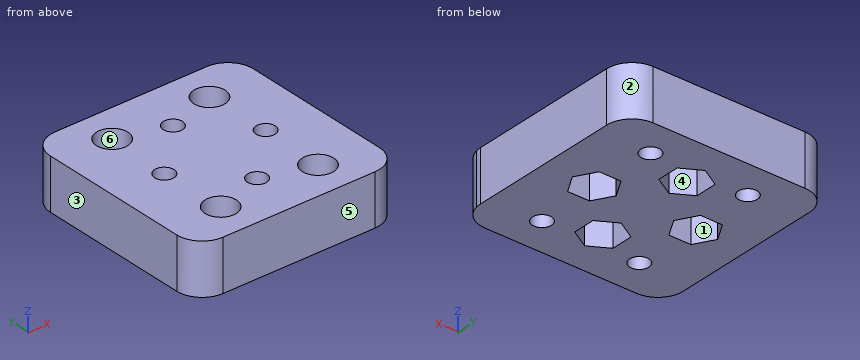
```python
from build123d import *

# Parameters (mm, degrees)
SKETCH1_W           = 50.8
SKETCH1_H           = 50.8
SKETCH1_R           = 2.413
BOSS_EXTRUDE1_DEPTH = 12.7
SKETCH2_R           = 2.413
CUT_EXTRUDE2_DEPTH  = 12.7
SKETCH7_R           = 2.413
CUT_EXTRUDE5_DEPTH  = 6.35
CUT_EXTRUDE6_DEPTH  = 73.955945611
SKETCH13_R          = 3.937
CUT_EXTRUDE7_DEPTH  = 4.826


with BuildPart() as part:
    # Sketch1 → Boss-Extrude1 (new body)
    with BuildSketch(Plane.XY):
        with Locations((25.4, -25.4)):
            Rectangle(SKETCH1_W, SKETCH1_H)
        with Locations((13.219909227, -9.017)):
            Circle(SKETCH1_R, mode=Mode.SUBTRACT)
        with Locations((37.603909227, -9.017)):
            Circle(SKETCH1_R, mode=Mode.SUBTRACT)
        with Locations((13.219909227, -41.783)):
            Circle(SKETCH1_R, mode=Mode.SUBTRACT)
        with Locations((37.603909227, -41.783)):
            Circle(SKETCH1_R, mode=Mode.SUBTRACT)
    extrude(amount=BOSS_EXTRUDE1_DEPTH)

    # Sketch2 → Cut-Extrude2 (cut)
    with BuildSketch(Plane(origin=(0, 0, 0), x_dir=(-1, 0, 0), z_dir=(0, 0, -1))):
        with Locations((-38.1, -25.4)):
            Circle(SKETCH2_R)
        with Locations((-25.4, -12.7)):
            Circle(SKETCH2_R)
        with Locations((-25.4, -38.1)):
            Circle(SKETCH2_R)
        with Locations((-12.7, -25.4)):
            Circle(SKETCH2_R)
    extrude(amount=-CUT_EXTRUDE2_DEPTH, mode=Mode.SUBTRACT)

    # Sketch7 → Cut-Extrude5 (cut)
    # profile 1 of 4: a face of its own
    with BuildSketch(Plane(origin=(0, 0, 0), x_dir=(-1, 0, 0), z_dir=(0, 0, -1))):
        Polygon((-20.6375, -40.849630657), (-20.6375, -35.350369343), (-25.4, -32.600738686), (-30.1625, -35.350369343), (-30.1625, -40.849630657), (-25.4, -43.599261314), align=None)
        with Locations((-25.4, -38.1)):
            Circle(SKETCH7_R, mode=Mode.SUBTRACT)
    # profile 2 of 4: a face of its own
    with BuildSketch(Plane(origin=(0, 0, 0), x_dir=(-1, 0, 0), z_dir=(0, 0, -1))):
        Polygon((-40.849630657, -30.1625), (-35.350369343, -30.1625), (-32.600738686, -25.4), (-35.350369343, -20.6375), (-40.849630657, -20.6375), (-43.599261314, -25.4), align=None)
        with Locations((-38.1, -25.4)):
            Circle(SKETCH7_R, mode=Mode.SUBTRACT)
    # profile 3 of 4: a face of its own
    with BuildSketch(Plane(origin=(0, 0, 0), x_dir=(-1, 0, 0), z_dir=(0, 0, -1))):
        Polygon((-9.950369343, -20.6375), (-15.449630657, -20.6375), (-18.199261314, -25.4), (-15.449630657, -30.1625), (-9.950369343, -30.1625), (-7.200738686, -25.4), align=None)
        with Locations((-12.7, -25.4)):
            Circle(SKETCH7_R, mode=Mode.SUBTRACT)
    # profile 4 of 4: a face of its own
    with BuildSketch(Plane(origin=(0, 0, 0), x_dir=(-1, 0, 0), z_dir=(0, 0, -1))):
        Polygon((-30.1625, -9.950369343), (-30.1625, -15.449630657), (-25.4, -18.199261314), (-20.6375, -15.449630657), (-20.6375, -9.950369343), (-25.4, -7.200738686), align=None)
        with Locations((-25.4, -12.7)):
            Circle(SKETCH7_R, mode=Mode.SUBTRACT)
    extrude(amount=-CUT_EXTRUDE5_DEPTH, mode=Mode.SUBTRACT)

    # Sketch10 → Cut-Extrude6 (cut, through all)
    with BuildSketch(Plane(origin=(0, 0, 0), x_dir=(-1, 0, 0), z_dir=(0, 0, -1))):
        with BuildLine():
            ThreePointArc((-50.8, -6.35), (-48.940128061, -1.859871939), (-44.45, 0))
            Line((-44.45, 0), (-50.8, 0))
            Line((-50.8, 0), (-50.8, -6.35))
        make_face()
        with BuildLine():
            Line((0, 0), (-6.35, 0))
            ThreePointArc((-6.35, 0), (-1.859871939, -1.859871939), (0, -6.35))
            Line((0, -6.35), (0, 0))
        make_face()
        with BuildLine():
            Line((0, -50.8), (0, -44.45))
            ThreePointArc((0, -44.45), (-1.859871939, -48.940128061), (-6.35, -50.8))
            Line((-6.35, -50.8), (0, -50.8))
        make_face()
        with BuildLine():
            ThreePointArc((-50.649504621, -45.824278884), (-50.762264029, -45.141247299), (-50.8, -44.45))
            Line((-50.8, -44.45), (-50.8, -50.8))
            Line((-50.8, -50.8), (-44.45, -50.8))
            ThreePointArc((-44.45, -50.8), (-48.424659047, -49.402230352), (-50.649504621, -45.824278884))
        make_face()
    extrude(amount=-CUT_EXTRUDE6_DEPTH, mode=Mode.SUBTRACT)

    # Sketch13 → Cut-Extrude7 (cut)
    with BuildSketch(Plane.XY.offset(12.7)):
        with Locations((37.603909227, -41.783)):
            Circle(SKETCH13_R)
        with Locations((13.219909227, -41.783)):
            Circle(SKETCH13_R)
        with Locations((37.603909227, -9.017)):
            Circle(SKETCH13_R)
        with Locations((13.219909227, -9.017)):
            Circle(SKETCH13_R)
    extrude(amount=-CUT_EXTRUDE7_DEPTH, mode=Mode.SUBTRACT)


solid = part.part
```
Input: part model. Units: mm. Frame: model coordinates. Face numbers are marked on the shaded views. A direction names the side the tool comes from. Coordinates: 2 decimals unless noted, no trailing zeros. Loops run counter-clockwise (first coordinate to the right, second up) from the corner with the lowest first, then second, coordinate; pieces in that order, holes last. Notation, with made-up numbers: M 86,55 L 131,55 A30 ccw 131,88 Z; hole C -1.5,17 d9. An arc over 180 degrees is marked long. Answer in a Markdown table with one row per item.
1. First-contact query: pin 1 (7.5 mm diameter, centred on x = 25.4, y = -12.7, fed in from -Z); pin 2 (4 mm diameter, centred on x = 13.22, y = -9.02, fed in from +Z); pin 3 (4 mm diameter, centred on x = 12, y = -42.5, fed in from +Z). Flat tips, straight axial feed; report the tip coordinate or a pass-through.
Response:
| item | result |
|---|---|
| pin 1 | stops at z = 6.35 |
| pin 2 | passes through |
| pin 3 | stops at z = 7.87 |
2. Material intervals for line 1 (X direction, y = -35.5, z = 1.75); line 2 (Y direction, x = 16, z = 10.5); line 3 (Y direction, x = 12.7, z = 11.25), sorted ascending.
Response:
| item | result |
|---|---|
| line 1 | x = 0 to 20.64, 30.16 to 50.8 |
| line 2 | y = -50.8 to -44.57, -39 to -11.8, -6.23 to 0 |
| line 3 | y = -50.8 to -45.69, -37.88 to -27.81, -22.99 to -12.92, -5.11 to 0 |
3. Section D-D, the plane x = 38.1. Output: boundary loops of the cut face in (y, z).
Response:
| item | result |
|---|---|
| outline | M -50.8,0 L -44.14,0 L -44.14,7.87 L -45.69,7.87 L -45.69,12.7 L -50.8,12.7 Z; M -39.42,0 L -30.16,0 L -30.16,6.35 L -27.81,6.35 L -27.81,12.7 L -37.88,12.7 L -37.88,7.87 L -39.42,7.87 Z; M -22.99,6.35 L -20.64,6.35 L -20.64,0 L -11.38,0 L -11.38,7.87 L -12.92,7.87 L -12.92,12.7 L -22.99,12.7 Z; M -6.66,0 L 0,0 L 0,12.7 L -5.11,12.7 L -5.11,7.87 L -6.66,7.87 Z |
4. Section A-A, the plane z = 10.5. Count the separate pieces of the cut face and the enclosed holes in it, then the cut area to 3 significant figures.
Response:
| item | result |
|---|---|
| separate pieces | 1 |
| enclosed holes | 8 |
| area | 2,280 mm2 |
5. Draft query along Y for the marked faces 1, 2 and 3. Return one class per face: pulls with the +Y half, pulls with the -Y half, needs draft (parallel to the pull), parting line crosses it, or undercut.
Response:
| item | result |
|---|---|
| face 1 | undercut |
| face 2 | pulls with the +Y half |
| face 3 | needs draft |
6. Reachability of the marked faces 4, 5 and 6 from +Z, -Z, +X, -X, +Y, -Y: full face, straight path, thin tool, end or side. Return the list, or none.
Response:
| item | result |
|---|---|
| face 4 | -Z |
| face 5 | +Z, -Z, +X, -X, -Y |
| face 6 | +Z |
7. Section C-C, the plane x = 12.7. Output: boundary loops of the cut face in (y, z).
Response:
| item | result |
|---|---|
| outline | M -50.8,0 L -44.14,0 L -44.14,7.87 L -45.69,7.87 L -45.69,12.7 L -50.8,12.7 Z; M -39.43,0 L -30.16,0 L -30.16,6.35 L -27.81,6.35 L -27.81,12.7 L -37.88,12.7 L -37.88,7.87 L -39.43,7.87 Z; M -22.99,6.35 L -20.64,6.35 L -20.64,0 L -11.37,0 L -11.37,7.87 L -12.92,7.87 L -12.92,12.7 L -22.99,12.7 Z; M -6.66,0 L 0,0 L 0,12.7 L -5.11,12.7 L -5.11,7.87 L -6.66,7.87 Z |
8. Section B-B, the plane y = -36.5. Output: boundary loops of the cut face in (x, z), then the cut area to 3 significant figures.
Response:
| item | result |
|---|---|
| outline | M 0,0 L 20.64,0 L 20.64,6.35 L 23.59,6.35 L 23.59,12.7 L 0,12.7 Z; M 27.21,6.35 L 30.16,6.35 L 30.16,0 L 50.8,0 L 50.8,12.7 L 27.21,12.7 Z |
| area | 562 mm2 |
